For this review, take the finished solid that the model builds, in its own axes (mm). Face numbers are marked on the shaded views. Round coordinates to 2 decimals unless told otherwise and drop trailing zeros. Order: outer loops, then holes, each group sorted by start corner. A loop starts at its lowest first (then second) coordinate and runs counter-clockwise, first axis right, second up. Notation, with made-up numbers: (-35, 71) - (17, 71) arc R3 cw to (17, 75) - close; hole circle Ø10 at (0.5, 46). An arc over 180 degrees is marked (long way). Write each question's results on one line, items separated by ' | '. Start each with the question number.
(1) Take a section at A-A, the plane z = 4.65. Give the boundary of the cut face in (x, y), plus the area to 3 significant figures.
(2) Draft analysis for pull direction Y (two halves, no side actions). For the marked faces 1 and 2, state which applies: pulls with the +Y half, pulls with the -Y half, needs draft (parallel to the pull), parting line crosses it, or undercut.
(3) Insertion check: pin 1 Ø1.5 at (y, z) = (-2.5, 3.5) entering from -X; pin 2 Ø2 at (x, z) = (-5.5, 4) entering from -Y; pin 3 Ø2 at (y, z) = (-2, 2.5) entering from +X; pin 4 Ø3.5 at (x, y) = (19.05, 0) entering from +Z. Each pin has a flat end and moves straight along its axis. Give the tip position at first contact, or say it passes through.
(4) Take a section at D-D, the plane x = 27. Give the boundary of the cut face in (y, z).
(5) For L1, parallel to Y at x = -6.35, z = 1.8; L2, parallel to Y at x = 19.05, z = 4.3; L3, parallel to X at y = -0.75, z = 2.3, list the stretches that pass through material, from the lowest coordinate up. Write a range as from..to.
(6) Take a section at B-B, the plane x = -6.35. Give the boundary of the cut face in (y, z).
(7) Take a section at C-C, the plane y = 0. Give the number of separate pieces and of enclosed holes in the cut face, plus the area to 3 significant figures.
```python
from build123d import *

# Parameters (mm, degrees)
F0_R     = 4.524375
F1_DEPTH = 2.38125
F0_R_2   = 1.984375
F0_R_3   = 2.976563
F2_DEPTH = 5.55625


with BuildPart() as f1:
    # F0 (on Top) → F1 (new body)
    with BuildSketch(Plane.XY):
        with BuildLine():
            ThreePointArc((-19.05, 8.89), (-27.94, 0), (-19.05, -8.89))
            Line((-19.05, -8.89), (44.45, -8.89))
            ThreePointArc((44.45, -8.89), (53.34, 0), (44.45, 8.89))
            Line((44.45, 8.89), (-19.05, 8.89))
        make_face()
        with Locations((-19.05, 0)):
            Circle(F0_R, mode=Mode.SUBTRACT)
        with Locations((-6.35, 0)):
            Circle(F0_R, mode=Mode.SUBTRACT)
        with Locations((19.05, 0)):
            Circle(F0_R, mode=Mode.SUBTRACT)
        with Locations((44.45, 0)):
            Circle(F0_R, mode=Mode.SUBTRACT)
    extrude(amount=F1_DEPTH)

    # F0 (on Top) → F2 (join)
    with BuildSketch(Plane.XY):
        with Locations((-19.05, 0)):
            Circle(F0_R)
        with Locations((-19.05, 0)):
            Circle(F0_R_2, mode=Mode.SUBTRACT)
        with Locations((-6.35, 0)):
            Circle(F0_R)
        with Locations((-6.35, 0)):
            Circle(F0_R_3, mode=Mode.SUBTRACT)
        with Locations((19.05, 0)):
            Circle(F0_R)
        with Locations((19.05, 0)):
            Circle(F0_R_3, mode=Mode.SUBTRACT)
        with Locations((44.45, 0)):
            Circle(F0_R)
        with Locations((44.45, 0)):
            Circle(F0_R_2, mode=Mode.SUBTRACT)
    extrude(amount=F2_DEPTH)


solid = f1.part
```
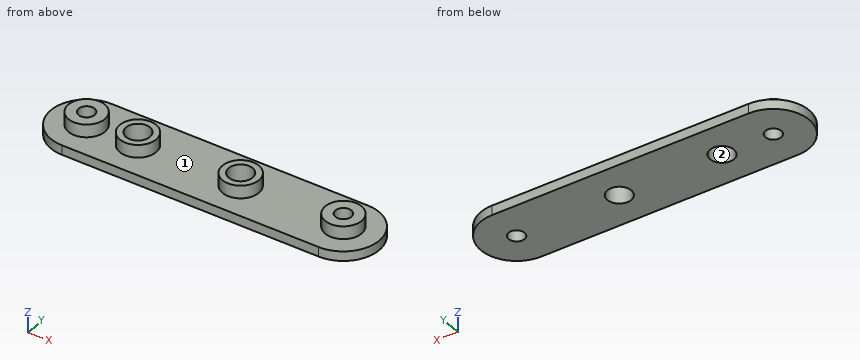
Results below:
1) outline: circle Ø9.05 at (-19.05, 0); circle Ø9.05 at (-6.35, 0); circle Ø9.05 at (19.05, 0); circle Ø9.05 at (44.45, 0); hole circle Ø3.97 at (-19.05, 0); hole circle Ø5.95 at (-6.35, 0); hole circle Ø5.95 at (19.05, 0); hole circle Ø3.97 at (44.45, 0) | area: 177 mm^2
2) face 1: needs draft | face 2: undercut
3) pin 1: stops at x = -23.22 | pin 2: stops at y = -4.52 | pin 3: stops at x = 53.28 | pin 4: passes through
4) outline: (-8.89, 0) - (8.89, 0) - (8.89, 2.38) - (-8.89, 2.38) - close
5) L1: y = -8.89..-2.98, 2.98..8.89 | L2: y = -4.52..-2.98, 2.98..4.52 | L3: x = -27.91..-20.89, -17.21..-9.23, -3.47..16.17, 21.93..42.61, 46.29..53.31
6) outline: (-8.89, 0) - (-2.98, 0) - (-2.98, 5.56) - (-4.52, 5.56) - (-4.52, 2.38) - (-8.89, 2.38) - close; (2.98, 0) - (8.89, 0) - (8.89, 2.38) - (4.52, 2.38) - (4.52, 5.56) - (2.98, 5.56) - close
7) separate pieces: 5 | enclosed holes: 0 | area: 198 mm^2
